Can you work these out from the model? Positions are in its coordinate system, mm. Give positions to 0.01 mm unless a question says otherwise; leave off trailing zeros. Order: outer loops, then holes, each group sorted by start corner. A loop starts at its lowest first (then second) coordinate and runs counter-clockwise, first axis right, second up. Notation, with made-up numbers: M 78,86 L 87,86 A12 ccw 87,105 Z; hole C 68.5,43 d4. An arc over 180 degrees is marked long. Answer as a JSON object with one key per item and string values.
```python
from build123d import *

# Parameters (mm, degrees)
SKETCH_1_R          = 21.345
EXTRUDE_1_DEPTH     = 8
SKETCH_2_R          = 4
CUT_EXTRUDE_1_DEPTH = 8
SKETCH_3_R          = 2.1
CUT_EXTRUDE_2_DEPTH = 8


with BuildPart() as part:
    # 스케치1 → 보스-돌출1 (new body)
    with BuildSketch(Plane(origin=(0, 0, 0), x_dir=(1, 0, 0), z_dir=(0, 1, 0))):
        Circle(SKETCH_1_R)
    extrude(amount=EXTRUDE_1_DEPTH)

    # 스케치2 → 컷-돌출1 (cut)
    with BuildSketch(Plane(origin=(0, 8, 0), x_dir=(1, 0, 0), z_dir=(0, 1, 0))):
        Circle(SKETCH_2_R)
    extrude(amount=-CUT_EXTRUDE_1_DEPTH, mode=Mode.SUBTRACT)

    # 스케치3 → 컷-돌출2 (cut)
    with BuildSketch(Plane(origin=(0, 8, 0), x_dir=(1, 0, 0), z_dir=(0, 1, 0))):
        with Locations((0, 8)):
            Circle(SKETCH_3_R)
        with Locations((0, 16)):
            Circle(SKETCH_3_R)
        with Locations((16, 0)):
            Circle(SKETCH_3_R)
        with Locations((8, 0)):
            Circle(SKETCH_3_R)
        with Locations((-8, 0)):
            Circle(SKETCH_3_R)
        with Locations((-16, 0)):
            Circle(SKETCH_3_R)
        with Locations((0, -8)):
            Circle(SKETCH_3_R)
        with Locations((0, -16)):
            Circle(SKETCH_3_R)
    extrude(amount=-CUT_EXTRUDE_2_DEPTH, mode=Mode.SUBTRACT)


solid = part.part
```
1) I need wall thicknesses on L1, parallel to X at y = 3, z = 0 (3 decimals); L2, parallel to Z at x = -16, y = 4.5; L3, parallel to X at y = 2.75, z = 6.5. Which ranges of each line are inside material? Lowest first, please.
Results found:
{"L1": "x = -21.345 to -18.1, -13.9 to -10.1, -5.9 to -4, 4 to 5.9, 10.1 to 13.9, 18.1 to 21.345", "L2": "z = -14.13 to -2.1, 2.1 to 14.13", "L3": "x = -20.33 to -1.47, 1.47 to 20.33"}
2) I want a section at C-C on y = 1.75. Count the separate pieces of the cut face and the enclosed holes in it, and give its area (3 significant figures).
Results found:
{"separate pieces": "1", "enclosed holes": "9", "area": "1,270 mm²"}
3) Thinking about a two-plate mould opening in X: for faces 1 (the face through (20.36, 3.94, -6.41)), 2 (the face through (13.9, 4.06, -0.09)), 3 (the face through (-0.3, 0, 4.4)), which applies, pulls with the +X half, pulls with the -X half, needs draft (parallel to the pull), parting line crosses it, or undercut?
Results found:
{"face 1": "parting line crosses it", "face 2": "undercut", "face 3": "needs draft"}
4) I want a section at B-B on z = 8. Write out the boundary of the cut face in (x, y), and give its area (3 significant figures).
Results found:
{"outline": "M -19.79,0 L -2.1,0 L -2.1,8 L -19.79,8 Z; M 2.1,0 L 19.79,0 L 19.79,8 L 2.1,8 Z", "area": "283 mm²"}
5) I want a section at D-D on x = 11. Write out the boundary of the cut face in (y, z).
Results found:
{"outline": "M 0,-18.29 L 8,-18.29 L 8,18.29 L 0,18.29 Z"}
6) I want a section at A-A on x = -8. Write out the boundary of the cut face in (y, z).
Results found:
{"outline": "M 0,-19.79 L 8,-19.79 L 8,-2.1 L 0,-2.1 Z; M 0,2.1 L 8,2.1 L 8,19.79 L 0,19.79 Z"}
